Input: part model. Units: mm. Frame: model coordinates. A direction names the side the tool comes from. Coordinates: 2 decimals unless noted, no trailing zeros. Write each loop counter-clockwise with the first axis right and the second up, starting at its lowest first coordinate (ties: lowest second). Pieces come first, ordered by that corner, then holes. Notation, with made-up numbers: (50.5, 75) -> (107.5, 75) arc R27 cw to (107.5, 111) -> close; hole circle Ø4 at (74, 54). An arc over 180 degrees is marked (long way). Use one line per item in the form item = value. Start each with the question number.
(1) Cut plane B-B on z = -8.5. Return the cut outline in (x, y).
(2) Ray query, line 1 along Y through (x, z) = (46.5, -8.5); line 2 along X through (y, z) = (-10, -3.5); line 3 along Z through (x, y) = (59.5, -11). Return the intervals inside material, ascending.
(3) Set-up query: faces 4 (the face through (67.92, -46, 1)), 5 (the face through (71, -65, -21)), 6 (the face through (44, -24, 0)). Return all of +Z, -Z, +X, -X, +Y, -Y with unobstructed straight access to the full face (end or side cutting, diameter ignored); none if empty.
(4) Cut plane D-D on x = 11. Return the cut outline in (y, z), plus the area to 3 significant figures.
(5) First-contact query: pin 1 (0.6 mm diameter, centred on y = 1, z = -9, fed in from +X). Flat tip, straight axial feed; report the tip coordinate or a pass-through.
(6) Cut plane A-A on y = -20.5. Return the cut outline in (x, z), plus the area to 3 significant figures.
(7) Cut plane C-C on y = -49.5. Return the cut outline in (x, z), plus the area to 3 significant figures.
(8) Pull-direction query (X, two-part tool) for faces 1 (the face through (36, -27.94, 1)), 2 (the face through (2, 1, -21)), 3 (the face through (74.4, -65.43, -9.15)); classes: released by +X, released by -X, zero draft, split by the parting line, or undercut.
```python
from build123d import *

# Parameters (mm, degrees)
SKETCH_1_W               = 73
SKETCH_1_H               = 64
SKETCH_1_W_2             = 22.86
SKETCH_1_H_2             = 10.16
SKETCH_1_W_3             = 12.7
SKETCH_1_H_3             = 20.32
SKETCH_1_W_4             = 19.66
SKETCH_1_H_4             = 35.56
SKETCH_1_W_5             = 17.78
SKETCH_1_H_5             = 25.4
EXTRUDE_1_DEPTH          = 2
SKETCH_2_W               = 77
SKETCH_2_H               = 68
SKETCH_2_W_2             = 73
SKETCH_2_H_2             = 64
EXTRUDE_2_DEPTH          = 25
FILLET_1_R               = 2
SKETCH_5_W               = 3
SKETCH_5_H               = 68
CUT_EXTRUDE_1_DEPTH      = 4
CUT_EXTRUDE_2_DEPTH      = 2
CUT_EXTRUDE_2_DEPTH_BACK = 2
SKETCH_7_W               = 3
SKETCH_7_H               = 68
SKETCH_8_W               = 20
SKETCH_8_H               = 15
CUT_EXTRUDE_3_DEPTH      = 2
SKETCH_9_W               = 15
SKETCH_9_H               = 13
CUT_EXTRUDE_4_DEPTH      = 2
SKETCH_10_W              = 12.7
SKETCH_10_H              = 6.7
CUT_EXTRUDE_5_DEPTH      = 2
EXTRUDE_3_DEPTH          = 5


with BuildPart() as part:
    # 草图1 → 凸台-拉伸1 (new body)
    with BuildSketch(Plane.XY):
        with Locations((36.5, -32)):
            Rectangle(SKETCH_1_W, SKETCH_1_H)
        with Locations((36.17, -10.16)):
            Rectangle(SKETCH_1_W_2, SKETCH_1_H_2, mode=Mode.SUBTRACT)
        with Locations((61.57, -22.86)):
            Rectangle(SKETCH_1_W_3, SKETCH_1_H_3, mode=Mode.SUBTRACT)
        with Locations((61.57, -45.72)):
            Rectangle(SKETCH_1_W_3, SKETCH_1_H_3, mode=Mode.SUBTRACT)
        with Locations((12.37, -33.02)):
            Rectangle(SKETCH_1_W_4, SKETCH_1_H_4, mode=Mode.SUBTRACT)
        with Locations((36.17, -40.64)):
            Rectangle(SKETCH_1_W_5, SKETCH_1_H_5, mode=Mode.SUBTRACT)
    extrude(amount=EXTRUDE_1_DEPTH)

    # 草图2 → 凸台-拉伸2 (add)
    with BuildSketch(Plane.XY.offset(2)):
        with Locations((36.5, -32)):
            Rectangle(SKETCH_2_W, SKETCH_2_H)
        with Locations((36.5, -32)):
            Rectangle(SKETCH_2_W_2, SKETCH_2_H_2, mode=Mode.SUBTRACT)
    extrude(amount=-EXTRUDE_2_DEPTH)

    # 圆角1
    fillet_1_edges = [part.edges().sort_by_distance(p)[0] for p in [
        (-2, 2, -10.5),
        (75, 2, -10.5),
        (75, -66, -10.5),
        (-2, -66, -10.5),
    ]]
    fillet(fillet_1_edges, radius=FILLET_1_R)

    # 草图5 → 切除-拉伸1 (cut)
    with BuildSketch(Plane(origin=(75, 0, 0), x_dir=(0, 0, -1), z_dir=(1, 0, 0))):
        with Locations((21.5, -32)):
            Rectangle(SKETCH_5_W, SKETCH_5_H)
    extrude(amount=-CUT_EXTRUDE_1_DEPTH, mode=Mode.SUBTRACT)

    # 草图7 → 切除-拉伸2 (cut, two sides: drawn at the far end of the back side and taken through both)
    with BuildSketch(Plane(origin=(0, 0, 0), x_dir=(0, 0, -1), z_dir=(1, 0, 0)).offset(-CUT_EXTRUDE_2_DEPTH_BACK)):
        with Locations((21.5, -32)):
            Rectangle(SKETCH_7_W, SKETCH_7_H)
    extrude(amount=CUT_EXTRUDE_2_DEPTH + CUT_EXTRUDE_2_DEPTH_BACK, mode=Mode.SUBTRACT)

    # 草图8 → 切除-拉伸3 (cut)
    with BuildSketch(Plane.XZ.offset(66)):
        with Locations((36, -5.5)):
            Rectangle(SKETCH_8_W, SKETCH_8_H)
    extrude(amount=-CUT_EXTRUDE_3_DEPTH, mode=Mode.SUBTRACT)

    # 草图9 → 切除-拉伸4 (cut)
    with BuildSketch(Plane(origin=(0, 2, 0), x_dir=(1, 0, 0), z_dir=(0, 1, 0))):
        with Locations((62.5, 9.5)):
            Rectangle(SKETCH_9_W, SKETCH_9_H)
    extrude(amount=-CUT_EXTRUDE_4_DEPTH, mode=Mode.SUBTRACT)

    # 草图10 → 切除-拉伸5 (cut)
    with BuildSketch(Plane.XY.offset(2)):
        with Locations((61.57, -5.35)):
            Rectangle(SKETCH_10_W, SKETCH_10_H)
    extrude(amount=-CUT_EXTRUDE_5_DEPTH, mode=Mode.SUBTRACT)

    # 草图12 → 凸台-拉伸3 (add)
    with BuildSketch(Plane(origin=(0, 0, 0), x_dir=(-1, 0, 0), z_dir=(0, 0, -1))):
        with BuildLine():
            Line((-1.5, -64), (0, -64))
            Line((0, -64), (0, -62.5))
            ThreePointArc((0, -62.5), (-2.560660172, -61.439339828), (-1.5, -64))
        make_face()
        with BuildLine():
            Line((-73, -64), (-73, -62.5))
            ThreePointArc((-73, -62.5), (-70.439339828, -61.439339828), (-71.5, -64))
            Line((-71.5, -64), (-73, -64))
        make_face()
        with BuildLine():
            Line((-71.5, 0), (-73, 0))
            Line((-73, 0), (-73, -1.5))
            ThreePointArc((-73, -1.5), (-70.439339828, -2.560660172), (-71.5, 0))
        make_face()
        with BuildLine():
            Line((0, 0), (0, -1.5))
            ThreePointArc((0, -1.5), (-2.560660172, -2.560660172), (-1.5, 0))
            Line((-1.5, 0), (0, 0))
        make_face()
    extrude(amount=EXTRUDE_3_DEPTH)


solid = part.part
```
Values:
q1.outline = (-2, -64) arc R2 ccw to (0, -66) -> (26, -66) -> (26, -64) -> (0, -64) -> (0, 0) -> (55, 0) -> (55, 2) -> (0, 2) arc R2 ccw to (-2, 0) -> close; (46, -66) -> (73, -66) arc R2 ccw to (75, -64) -> (75, 0) arc R2 ccw to (73, 2) -> (70, 2) -> (70, 0) -> (73, 0) -> (73, -64) -> (46, -64) -> close
q2.line_1 = -66 to -64, 0 to 2
q2.line_2 = -2 to 0, 73 to 75
q2.line_3 = 0 to 2
q3.face_4 = +Z, -Z
q3.face_5 = -Z, +X, +Y, -Y
q3.face_6 = -Z
q4.outline = (-66, -23) -> (-64, -23) -> (-64, 0) -> (-50.8, 0) -> (-50.8, 2) -> (-66, 2) -> close; (-15.24, 0) -> (0, 0) -> (0, -23) -> (2, -23) -> (2, 2) -> (-15.24, 2) -> close
q4.area = 157 mm2
q5.pin_1 = 74.87
q6.outline = (-2, -20) -> (0, -20) -> (0, 0) -> (2.54, 0) -> (2.54, 2) -> (-2, 2) -> close; (22.2, 0) -> (55.22, 0) -> (55.22, 2) -> (22.2, 2) -> close; (67.92, 0) -> (73, 0) -> (73, -20) -> (75, -20) -> (75, 2) -> (67.92, 2) -> close
q6.area = 169 mm2
q7.outline = (-2, -20) -> (0, -20) -> (0, 0) -> (2.54, 0) -> (2.54, 2) -> (-2, 2) -> close; (22.2, 0) -> (27.28, 0) -> (27.28, 2) -> (22.2, 2) -> close; (45.06, 0) -> (55.22, 0) -> (55.22, 2) -> (45.06, 2) -> close; (67.92, 0) -> (73, 0) -> (73, -20) -> (75, -20) -> (75, 2) -> (67.92, 2) -> close
q7.area = 134 mm2
q8.face_1 = undercut
q8.face_2 = released by -X
q8.face_3 = released by +X
